Geometry: see drawing. Coordinates: mm, zero at the bounding-box minimum. A direction names the side the tool comes from. Give positions to 0.01 mm unless a question says otherwise; leave off trailing zeros. Write each loop counter-clockwise with the first axis right and the second up, starting at its lowest first coordinate (ties: lowest second). Pieces come first, ordered by that corner, then holes. Notation, with made-up numbers: M 41.5,79.5 L 51.5,79.5 A19 cw 51.5,108.5 Z; hole C 51,-39 d7. An arc over 180 degrees is marked long. Use a Markdown table: item, result. Add a question column.
(1) Pin query (flat end, axial travel): pin 1 Ø7.5 at (x, y) = (24.63, 19.05) entering from -Z; pin 2 Ø5 at (x, y) = (24.63, 57.15) entering from +Z; pin 3 Ø1 at (y, z) = (7.5, 66.5) entering from +X; pin 4 Ø18.5 at (x, y) = (20.5, 31.5) entering from +Z. Return the tip coordinate at first contact, or that it passes through.
(2) Cut plane B-B (y = 25). Output: boundary loops of the cut face in (x, z).
(3) Cut plane A-A (y = 38.1). Output: boundary loops of the cut face in (x, z).
(4) Material intervals for L1, parallel to X at y = 38, z = 4; L2, parallel to Z at x = 16, y = 4.5, sorted ascending.
(5) Cut plane D-D (z = 61). Output: boundary loops of the cut face in (x, y), plus the area to 3 significant figures.
(6) Cut plane C-C (x = 16.5). Output: boundary loops of the cut face in (y, z).
(7) Reachability of the marked faces 1 and 2 from +Z, -Z, +X, -X, +Y, -Y: full face, straight path, thin tool, end or side. Return the list, or none.
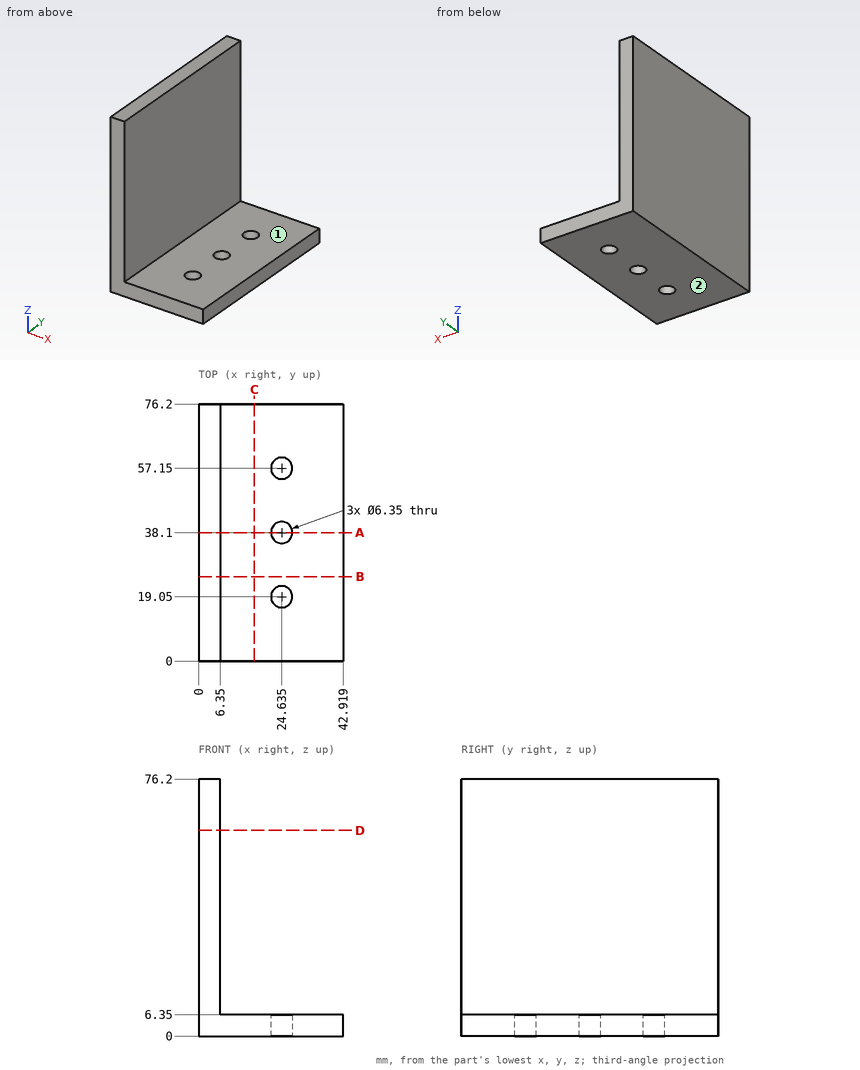
Answer list:
| question | item | result |
|---|---|---|
| 1 | pin 1 | z = 0 |
| 1 | pin 2 | through |
| 1 | pin 3 | x = 6.35 |
| 1 | pin 4 | z = 6.35 |
| 2 | outline | M 0,0 L 42.92,0 L 42.92,6.35 L 6.35,6.35 L 6.35,76.2 L 0,76.2 Z |
| 3 | outline | M 0,0 L 21.46,0 L 21.46,6.35 L 6.35,6.35 L 6.35,76.2 L 0,76.2 Z; M 27.81,0 L 42.92,0 L 42.92,6.35 L 27.81,6.35 Z |
| 4 | L1 | 0 to 21.46, 27.81 to 42.92 |
| 4 | L2 | 0 to 6.35 |
| 5 | outline | M 0,0 L 6.35,0 L 6.35,76.2 L 0,76.2 Z |
| 5 | area | 484 mm² |
| 6 | outline | M 0,0 L 76.2,0 L 76.2,6.35 L 0,6.35 Z |
| 7 | face 1 | +Z, +X, +Y, -Y |
| 7 | face 2 | -Z, +X, -X, +Y, -Y |
